The model under review builds one solid part; all positions refer to its coordinate system, in mm. Face numbers are marked on the shaded views. Round coordinates to 2 decimals unless told otherwise and drop trailing zeros. Loops run counter-clockwise (first coordinate to the right, second up) from the corner with the lowest first, then second, coordinate; pieces in that order, holes last. Notation, with made-up numbers: M 63.25,-7 L 84.25,-7 A15 ccw 84.25,19 Z; hole C 14.25,39 d3. An arc over 180 degrees is marked long. One line per question, with ' | ' between items.
from build123d import *

# Parameters (mm, degrees)
SKETCH1_R           = 165.1
BOSS_EXTRUDE1_DEPTH = 127
SKETCH2_R           = 76.2
CUT_EXTRUDE2_DEPTH  = 128
FILLET1_R           = 17.78
FILLET2_R           = 45.72


with BuildPart() as part:
    # Sketch1 → Boss-Extrude1 (new body)
    with BuildSketch(Plane(origin=(0, 0, 0), x_dir=(0, 0, -1), z_dir=(1, 0, 0))):
        Circle(SKETCH1_R)
    extrude(amount=BOSS_EXTRUDE1_DEPTH)

    # Sketch2 → Cut-Extrude2 (cut, through all)
    with BuildSketch(Plane(origin=(127, 0, 0), x_dir=(0, 0, -1), z_dir=(1, 0, 0))):
        Circle(SKETCH2_R)
    extrude(amount=-CUT_EXTRUDE2_DEPTH, mode=Mode.SUBTRACT)

    # Fillet1
    fillet1_edges = [part.edges().sort_by_distance(p)[0] for p in [
        (0, 0, 76.2),
        (127, 0, 76.2),
    ]]
    fillet(fillet1_edges, radius=FILLET1_R)

    # Fillet2
    fillet2_edges = [part.edges().sort_by_distance(p)[0] for p in [
        (0, 0, 165.1),
        (127, 0, 165.1),
    ]]
    fillet(fillet2_edges, radius=FILLET2_R)


solid = part.part
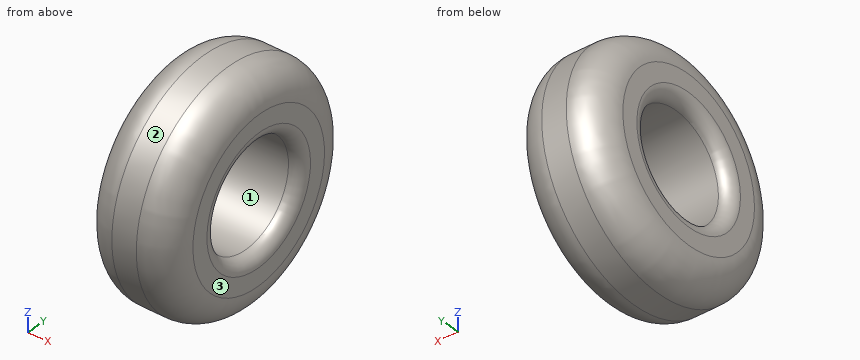
1) Insertion check: P1, Ø2, axis at x = 112, z = 28.5, coming from the -Y side; P2, Ø6, axis at x = 24.5, z = -64, coming from the +Y side; P3, Ø2, axis at x = 65, y = -63.5, coming from the +Z side. Each pin has a flat end and moves straight along its axis. Give the tip position at first contact, or say it passes through.
Output values:
P1: stops at y = -151.48 | P2: stops at y = 148.55 | P3: stops at z = 152.81
2) For line 1 (Y direction, x = 56, z = 0); line 2 (Y direction, x = 85, z = 0); line 3 (Z direction, x = 9.5, y = -21), list the stretches that pass through material, from the lowest coordinate up.
Output values:
line 1: y = -165.1 to -76.2, 76.2 to 165.1 | line 2: y = -164.95 to -76.2, 76.2 to 164.95 | line 3: z = -145.78 to -75.37, 75.37 to 145.78
3) Add section A-A on z = 0. State the section outline as (x, y) points.
Output values:
outline: M 0,-119.38 A45.72 ccw 45.72,-165.1 L 81.28,-165.1 A45.72 ccw 127,-119.38 L 127,-93.98 A17.78 ccw 109.22,-76.2 L 17.78,-76.2 A17.78 ccw 0,-93.98 Z; M 0,93.98 A17.78 ccw 17.78,76.2 L 109.22,76.2 A17.78 ccw 127,93.98 L 127,119.38 A45.72 ccw 81.28,165.1 L 45.72,165.1 A45.72 ccw 0,119.38 Z
4) Add section D-D on x = 35. State the section outline as (y, z) points, then the cut area to 3 significant figures.
Output values:
outline: C 0,0 d327.65; hole C 0,0 d152.4 | area: 66,100 mm²
5) Add section C-C on x = 93.5. State the section outline as (y, z) points, then the cut area to 3 significant figures.
Output values:
outline: C 0,0 d326.87; hole C 0,0 d152.4 | area: 65,700 mm²
6) Mouldability with a two-part tool opening along Z and no side actions: class the marked faces 1, 2 and 3 as +Z half, -Z half, draft (parallel to the pull), parting line (faces both ways), or undercut.
Output values:
face 1: undercut | face 2: parting line | face 3: draft
